Design review of the part built by this model. Coordinates are the model's own, in mm. Face numbers are marked on the shaded views. A direction names the side the tool comes from. Coordinates: 2 decimals unless noted, no trailing zeros. Loops run counter-clockwise (first coordinate to the right, second up) from the corner with the lowest first, then second, coordinate; pieces in that order, holes last. Notation, with made-up numbers: (-16, -40) -> (17, -40) arc R31 ccw to (17, -11) -> close; hole circle Ø11 at (68, 72.25). An arc over 180 degrees is marked (long way). Use a Markdown table: item, result. Add a question column.
Q1. Clearance check with flat-ended pins moving along their axes: pin 1 Ø1.5 at (x, y) = (17, -3.5) entering from +Z; pin 2 Ø6 at (y, z) = (3.5, 4) entering from -X; pin 3 Ø5 at (y, z) = (3, 1.5) entering from +X; pin 4 Ø1 at (x, z) = (-22, 6) entering from +Y. State where each tip first meets the part, or that it passes through.
Q2. Take a section at A-A on y = -2.5. Write out the cut boundary in (x, z).
Q3. Draft analysis for pull direction Y (two halves, no side actions). For the marked faces 1, 2 and 3, state which applies: pulls with the +Y half, pulls with the -Y half, needs draft (parallel to the pull), parting line crosses it, or undercut.
Q4. Take a section at D-D on y = 2.5. Write out the cut boundary in (x, z).
Q5. Take a section at C-C on z = 5.75. Write out the cut boundary in (x, y) (1 decimal), plus the area to 3 significant figures.
Q6. For the marked faces 4 and 5, list the 3-axis set-ups (+Z, -Z, +X, -X, +Y, -Y) from which the entire face can be reached by the end or side of a thin tool; tool diameter is ignored.
Q7. For probe 1 along X at (y, z) = (4.5, 5.75); probe 2 along X at (y, z) = (-2, 9.25); probe 3 along Y at (x, z) = (-3.5, 7), list the stretches that pass through material, from the lowest coordinate up.
Q8. Take a section at B-B on x = 10.5. Write out the cut boundary in (y, z).
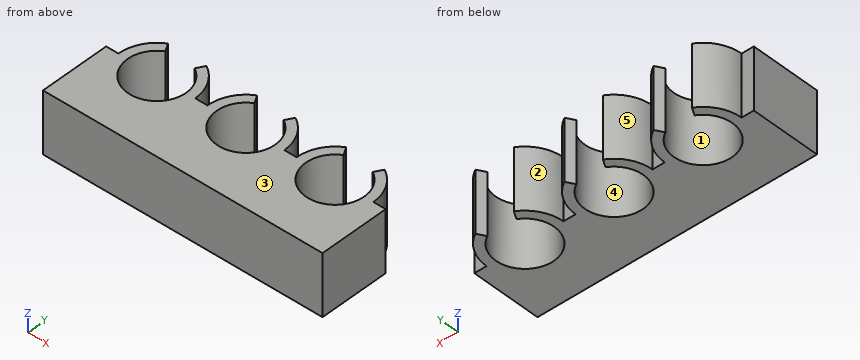
from build123d import *

# Parameters (mm, degrees)
BOSS_EXTRUDE1_DEPTH = 10


with BuildPart() as part:
    # Sketch4 → Boss-Extrude1 (new body)
    with BuildSketch(Plane.XY):
        with BuildLine():
            Line((-20.7875, 0), (-22.7875, 0))
            Line((-22.7875, 0), (-22.7875, -11.2625))
            Line((-22.7875, -11.2625), (22.7875, -11.2625))
            Line((22.7875, -11.2625), (22.7875, 0))
            Line((22.7875, 0), (20.7875, 0))
            ThreePointArc((20.7875, 0), (19.948484091, 3.13125), (17.65625, 5.423484091))
            Line((17.65625, 5.423484091), (16.90625, 4.124445986))
            ThreePointArc((16.90625, 4.124445986), (14.525, -4.7625), (12.14375, 4.124445986))
            Line((12.14375, 4.124445986), (11.39375, 5.423484091))
            ThreePointArc((11.39375, 5.423484091), (9.101515909, 3.13125), (8.2625, 0))
            Line((8.2625, 0), (6.2625, 0))
            ThreePointArc((6.2625, 0), (5.423484091, 3.13125), (3.13125, 5.423484091))
            Line((3.13125, 5.423484091), (2.38125, 4.124445986))
            ThreePointArc((2.38125, 4.124445986), (0, -4.7625), (-2.38125, 4.124445986))
            Line((-2.38125, 4.124445986), (-3.13125, 5.423484091))
            ThreePointArc((-3.13125, 5.423484091), (-5.423484091, 3.13125), (-6.2625, 0))
            Line((-6.2625, 0), (-8.2625, 0))
            ThreePointArc((-8.2625, 0), (-9.101515909, 3.13125), (-11.39375, 5.423484091))
            Line((-11.39375, 5.423484091), (-12.14375, 4.124445986))
            ThreePointArc((-12.14375, 4.124445986), (-14.525, -4.7625), (-16.90625, 4.124445986))
            Line((-16.90625, 4.124445986), (-17.65625, 5.423484091))
            ThreePointArc((-17.65625, 5.423484091), (-19.948484091, 3.13125), (-20.7875, 0))
        make_face()
    extrude(amount=BOSS_EXTRUDE1_DEPTH)


solid = part.part
Answer list:
| question | item | result |
|---|---|---|
| 1 | pin 1 | z = 10 |
| 1 | pin 2 | x = -20.77 |
| 1 | pin 3 | x = 20.77 |
| 1 | pin 4 | y = 0 |
| 2 | outline | (-22.79, 0) -> (-18.58, 0) -> (-18.58, 10) -> (-22.79, 10) -> close; (-10.47, 0) -> (-4.05, 0) -> (-4.05, 10) -> (-10.47, 10) -> close; (4.05, 0) -> (10.47, 0) -> (10.47, 10) -> (4.05, 10) -> close; (18.58, 0) -> (22.79, 0) -> (22.79, 10) -> (18.58, 10) -> close |
| 3 | face 1 | undercut |
| 3 | face 2 | pulls with the +Y half |
| 3 | face 3 | needs draft |
| 4 | outline | (-20.27, 0) -> (-18.58, 0) -> (-18.58, 10) -> (-20.27, 10) -> close; (-10.47, 0) -> (-8.78, 0) -> (-8.78, 10) -> (-10.47, 10) -> close; (-5.74, 0) -> (-4.05, 0) -> (-4.05, 10) -> (-5.74, 10) -> close; (4.05, 0) -> (5.74, 0) -> (5.74, 10) -> (4.05, 10) -> close; (8.78, 0) -> (10.47, 0) -> (10.47, 10) -> (8.78, 10) -> close; (18.58, 0) -> (20.27, 0) -> (20.27, 10) -> (18.58, 10) -> close |
| 5 | outline | (-22.8, -11.3) -> (22.8, -11.3) -> (22.8, 0) -> (20.8, 0) arc R6.3 ccw to (17.7, 5.4) -> (16.9, 4.1) arc R4.8 cw (long way) to (12.1, 4.1) -> (11.4, 5.4) arc R6.3 ccw to (8.3, 0) -> (6.3, 0) arc R6.3 ccw to (3.1, 5.4) -> (2.4, 4.1) arc R4.8 cw (long way) to (-2.4, 4.1) -> (-3.1, 5.4) arc R6.3 ccw to (-6.3, 0) -> (-8.3, 0) arc R6.3 ccw to (-11.4, 5.4) -> (-12.1, 4.1) arc R4.8 cw (long way) to (-16.9, 4.1) -> (-17.7, 5.4) arc R6.3 ccw to (-20.8, 0) -> (-22.8, 0) -> close |
| 5 | area | 458 mm² |
| 6 | face 4 | +Z, -Z |
| 6 | face 5 | +Z, -Z, +Y |
| 7 | probe 1 | -18.88 to -17.12, -11.93 to -10.17, -4.36 to -2.6, 2.6 to 4.36, 10.17 to 11.93, 17.12 to 18.88 |
| 7 | probe 2 | -22.79 to -18.85, -10.2 to -4.32, 4.32 to 10.2, 18.85 to 22.79 |
| 7 | probe 3 | -11.26 to -3.23, 3.23 to 5.19 |
| 8 | outline | (-11.26, 0) -> (-2.55, 0) -> (-2.55, 10) -> (-11.26, 10) -> close; (2.55, 0) -> (4.8, 0) -> (4.8, 10) -> (2.55, 10) -> close |
